Autodesk Inventor part; units mm, degrees
ref_plane "YZ Plane" through (0, 0, 0) normal (1, 0, 0) x (0, 1, 0)
ref_plane "XZ Plane" through (0, 0, 0) normal (0, 1, 0) x (-1, 0, 0)
ref_plane "XY Plane" through (0, 0, 0) normal (0, 0, 1) x (1, 0, 0)
sketch "Sketch1" plane through (0, 0, 0) normal (0, 1, 0) x (-1, 0, 0)
  circle A0 centre (0, 0) radius 600
  line L0 (0, 0) -> (507.7952, 0) construction
  line L1 (507.7952, 0) -> (507.7952, -319.5997) construction
  line L2 (507.7952, 0) -> (507.7952, 319.5997) construction
  line L3 (507.7952, 319.5997) -> (507.7952, 269.5997)
  line L4 (507.7952, -319.5997) -> (507.7952, -269.5997)
  line L5 (507.7952, 319.5997) -> (727.7952, 319.5997)
  line L6 (507.7952, -319.5997) -> (727.7952, -319.5997)
  line L7 (757.7952, -289.5997) -> (757.7952, 289.5997)
  line L8 (707.7952, 239.5997) -> (707.7952, -239.5997)
  line L9 (507.7952, -269.5997) -> (677.7952, -269.5997)
  line L10 (507.7952, 269.5997) -> (677.7952, 269.5997)
  arc A1 (757.7952, 289.5997) -> (727.7952, 319.5997) centre (727.7952, 289.5997) ccw
  arc A2 (727.7952, -319.5997) -> (757.7952, -289.5997) centre (727.7952, -289.5997) ccw
  arc A3 (677.7952, -269.5997) -> (707.7952, -239.5997) centre (677.7952, -239.5997) ccw
  arc A4 (707.7952, 239.5997) -> (677.7952, 269.5997) centre (677.7952, 239.5997) ccw
  point P0 (757.7952, 319.5997)
  point P1 (707.7952, 319.5997)
  point P2 (707.7952, -319.5997)
  point P3 (536.0186, 269.5997)
  point P4 (536.0186, -269.5997)
  dimension "d0" = 1200
  dimension "d1" = 50
  dimension "d2" = 319.5997
  dimension "d3" = 50
  dimension "d4" = 250
  dimension "d7" = 50
  dimension "d8" = 30
  dimension "d9" = 30
  dimension "d10" = 30
  dimension "d11" = 30
extrude "Extrusion1" add sketch "Sketch1" along normal blind 25 contours L5 A1 L7 A2 L6 A0 L9 A3 L8 A4 L10
properties part number "handlebar"
CAD build for the part. Positions are in the model's coordinates, mm. A direction names the side the tool comes from. Round coordinates to 2 decimals unless told otherwise and drop trailing zeros. Write each loop counter-clockwise with the first axis right and the second up, starting at its lowest first coordinate (ties: lowest second). Pieces come first, ordered by that corner, then holes. Notation, with made-up numbers: M 87.5,26 L 97.5,26 A7 cw 97.5,31 Z; hole C -0.5,-21 d2. An arc over 180 degrees is marked long. Use a Markdown table: item, result. Add a question column.
1. Pull direction Z, two halves, no side cores. Call faces 3 (the face through (-757.795, 12, -4)), 4 (the face through (-616, 12, -319.6)), 5 (the face through (-522.3, 12.3, 295.3)): released by +Z, released by -Z, zero draft, split by the parting line, or undercut.
2. Slice it at B-B on y = 10. Give the cut face in (x, z), then the cut area to 3 significant figures.
3. Slice it at A-A on x = -596. Give the cut face in (y, z), then the cut area to 3 significant figures.
4. Slice it at C-C on z = 69. Give the cut face in (x, y), then the cut area to 3 significant figures.
5. Flat gauge pins, fed straight in: P1, Ø8, axis at y = 8, z = -95.5, coming from the +X side; P2, Ø10, axis at y = 15.5, z = 237.5, coming from the +X side. Where does each tip first touch, or does it go through?
6. Drill centre lines: probe 1 along Z at (x, y) = (-673.5, 19.5); probe 2 along Z at (x, y) = (-691.5, 23); probe 3 along X at (y, z) = (2.25, -92). Where is each one in solid material? Low to high.
7. Slice it at D-D on x = -686. Give the cut face in (y, z), then the cut area to 3 significant figures.
8. 3-axis set-ups, long thin cutter, end or side, ignore diameter. For faces 1 (the face through (-699.24, 12.32, -260.58)), 2 (the face through (-714, 25, 4)): which of +Z, -Z, +X, -X, +Y, -Y reach the whole face in a straight line?
Reply:
| question | item | result |
|---|---|---|
| 1 | face 3 | zero draft |
| 1 | face 4 | released by -Z |
| 1 | face 5 | undercut |
| 2 | outline | M -757.8,-289.6 A30 ccw -727.8,-319.6 L -507.8,-319.6 A600 cw -536.02,-269.6 L -677.8,-269.6 A30 cw -707.8,-239.6 L -707.8,239.6 A30 cw -677.8,269.6 L -536.02,269.6 A600 cw -507.8,319.6 L -727.8,319.6 A30 ccw -757.8,289.6 Z |
| 2 | area | 50,500 mm^2 |
| 3 | outline | M 0,-319.6 L 25,-319.6 L 25,-269.6 L 0,-269.6 Z; M 0,269.6 L 25,269.6 L 25,319.6 L 0,319.6 Z |
| 3 | area | 2,500 mm^2 |
| 4 | outline | M -757.8,0 L -707.8,0 L -707.8,25 L -757.8,25 Z |
| 4 | area | 1,250 mm^2 |
| 5 | P1 | stops at x = -707.8 |
| 5 | P2 | stops at x = -707.65 |
| 6 | probe 1 | z = -319.6 to -269.6, 269.6 to 319.6 |
| 6 | probe 2 | z = -319.6 to -266.29, 266.29 to 319.6 |
| 6 | probe 3 | x = -757.8 to -707.8 |
| 7 | outline | M 0,-319.6 L 25,-319.6 L 25,-268.46 L 0,-268.46 Z; M 0,268.46 L 25,268.46 L 25,319.6 L 0,319.6 Z |
| 7 | area | 2,560 mm^2 |
| 8 | face 1 | +X, +Y, -Y |
| 8 | face 2 | +Z, -Z, +X, -X, +Y |
